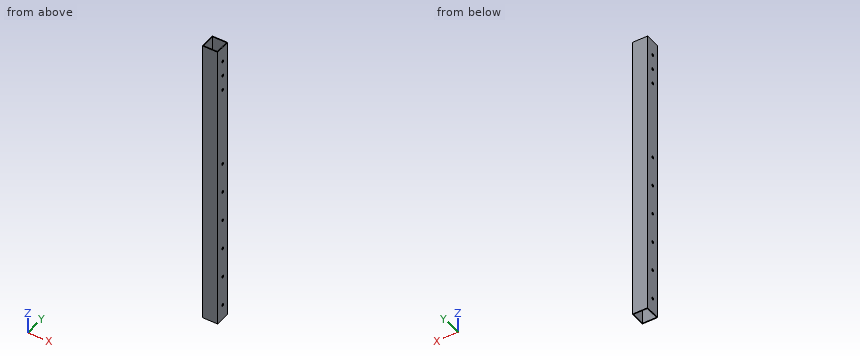
from build123d import *

# Parameters (mm, degrees)
F0_W     = 50
F0_H     = 50
F0_W_2   = 45
F0_H_2   = 45
F1_DEPTH = 962
F3_D     = 8.8


with BuildPart() as f1:
    # F0 (on Top) → F1 (new body)
    with BuildSketch(Plane.XY):
        Rectangle(F0_W, F0_H)
        Rectangle(F0_W_2, F0_H_2, mode=Mode.SUBTRACT)
    extrude(amount=F1_DEPTH)

    # F3 (through all)
    with Locations(Plane(origin=(-25, 0, 0), x_dir=(0, -1, 0), z_dir=(-1, 0, 0))):
        with Locations((0, 350), (0, 450), (0, 550), (0, 250), (0, 150), (0, 50), (0, 812), (0, 912), (0, 862)):
            Hole(F3_D / 2)


solid = f1.part
Could you check a few things on this model? Use its own coordinates, in mm. Coordinates: 2 decimals unless noted, no trailing zeros. Loops run counter-clockwise (first coordinate to the right, second up) from the corner with the lowest first, then second, coordinate; pieces in that order, holes last.
1. Imagine slicing it at B-B (x = 10). Please give me the cut outline in (y, z), and give its area (3 significant figures).
2. I need wall thicknesses on L1, parallel to X at y = 16, z = 611; L2, parallel to Y at x = 24.4, z = 912. Which ranges of each line are inside material? Lowest first, please.
3. Imagine slicing it at A-A (z = 221.5). Please give me the cut outline in (x, y).
Computed values:
1. outline: (-25, 0) - (-22.5, 0) - (-22.5, 962) - (-25, 962) - close; (22.5, 0) - (25, 0) - (25, 962) - (22.5, 962) - close
1. area: 4,810 mm2
2. L1: x = -25 to -22.5, 22.5 to 25
2. L2: y = -25 to -4.4, 4.4 to 25
3. outline: (-25, -25) - (25, -25) - (25, 25) - (-25, 25) - close; hole (-22.5, -22.5) - (22.5, -22.5) - (22.5, 22.5) - (-22.5, 22.5) - close
